Can you work these out from the model? Positions are in its coordinate system, mm. Face numbers are marked on the shaded views. A direction names the side the tool comes from. Coordinates: 2 decimals unless noted, no trailing zeros. Order: outer loops, then holes, each group sorted by start corner. A loop starts at its lowest first (then second) coordinate and runs counter-clockwise, first axis right, second up.
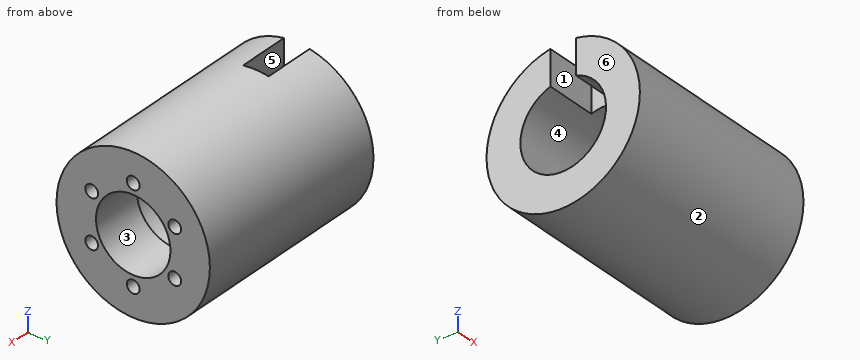
```python
from build123d import *

# Parameters (mm, degrees)
SKETCH1_W          = 25.4
SKETCH1_H          = 5.3975
SKETCH2_R          = 3.175
SKETCH2_R_2        = 18.5
CUT_EXTRUDE1_DEPTH = 25.4
CIRPATTERN1_COUNT  = 6
SKETCH3_W          = 25.4
SKETCH3_H          = 12.7
CUT_EXTRUDE2_DEPTH = 39.1


with BuildPart() as part:
    # Sketch1 → Revolve1 (revolve)
    with BuildSketch(Plane.XY):
        Polygon((-50.8, 38.1), (-50.8, 21.2725), (25.4, 21.2725), (50.8, 21.2725), (50.8, 38.1), (44.45, 38.1), align=None)
        with Locations((38.1, 18.57375)):
            Rectangle(SKETCH1_W, SKETCH1_H)
    revolve(axis=Axis((-50.8, 0, 0), (1, 0, 0)))

    # Sketch2 → Cut-Extrude1 (cut)
    with BuildSketch(Plane(origin=(50.8, 0, 0), x_dir=(0, 0, -1), z_dir=(1, 0, 0))):
        with Locations((-11.90625, -20.622229928)):
            Circle(SKETCH2_R)
        with Locations((11.90625, -20.622229928)):
            Circle(SKETCH2_R)
        with Locations((23.8125, 0)):
            Circle(SKETCH2_R)
        with Locations((11.90625, 20.622229928)):
            Circle(SKETCH2_R)
        with Locations((-11.90625, 20.622229928)):
            Circle(SKETCH2_R)
        Circle(SKETCH2_R_2)
    cut_extrude1 = extrude(amount=-CUT_EXTRUDE1_DEPTH, mode=Mode.SUBTRACT)

    # CirPattern1: Cut-Extrude1 ×6 about axis
    cirpattern1_axis = Axis((-50.8, 0, 0), (-1, 0, 0))
    for i in range(1, CIRPATTERN1_COUNT):
        add(cut_extrude1.rotate(cirpattern1_axis, i * 360 / CIRPATTERN1_COUNT), mode=Mode.SUBTRACT)

    # Sketch3 → Cut-Extrude2 (cut, through all)
    with BuildSketch(Plane.XY):
        with Locations((-38.1, 0)):
            Rectangle(SKETCH3_W, SKETCH3_H)
    extrude(amount=CUT_EXTRUDE2_DEPTH, mode=Mode.SUBTRACT)


solid = part.part
```
1. I'm going to push flat-ended pins straight in: pin 1 (10 mm diameter, centred on x = -33.5, z = 26, fed in from +Y); pin 2 (6 mm diameter, centred on x = -20, z = -6, fed in from -Y); pin 3 (8.5 mm diameter, centred on x = -40.5, z = 31, fed in from -Y). Where does each tip first touch, or does it pass through?
Completed:
pin 1: stops at y = 31.79
pin 2: stops at y = -37.98
pin 3: stops at y = -27.13
2. On a 3-axis mill with a long thin cutter (end or side, diameter ignored), from which of +Z, -Z, +X, -X, +Y, -Y can I reach the whole of each face in a straight line? I mean the marked faces 4, 5 and 6. Say none if no direction works.
Completed:
face 4: -X
face 5: +Z, -X
face 6: +Z, -Z, -X, +Y, -Y
3. Imagine slicing it at C-C on x = 45. Give the number of separate pieces and of enclosed holes in the cut face, then the cut area to 3 significant figures.
Completed:
separate pieces: 1
enclosed holes: 7
area: 3,300 mm2
4. Imagine slicing it at D-D on z = -16.5. Please give me the cut outline in (x, y).
Completed:
outline: (-50.8, -34.34) - (50.8, -34.34) - (50.8, -8.37) - (25.4, -8.37) - (25.4, -13.43) - (-50.8, -13.43) - close; (-50.8, 13.43) - (25.4, 13.43) - (25.4, 8.37) - (50.8, 8.37) - (50.8, 34.34) - (-50.8, 34.34) - close
5. Imagine slicing it at B-B on y = 0. Please give me the cut outline in (x, z).
Completed:
outline: (-50.8, -38.1) - (50.8, -38.1) - (50.8, -26.99) - (25.4, -26.99) - (25.4, -21.27) - (-50.8, -21.27) - close; (-25.4, 21.27) - (25.4, 21.27) - (25.4, 26.99) - (50.8, 26.99) - (50.8, 38.1) - (-25.4, 38.1) - close; (25.4, -20.64) - (50.8, -20.64) - (50.8, -18.5) - (25.4, -18.5) - close; (25.4, 18.5) - (50.8, 18.5) - (50.8, 20.64) - (25.4, 20.64) - close
6. Thinking about a two-plate mould opening in Z: for the marked faces 1, 2 and 3, which applies, pulls with the +Z half, pulls with the -Z half, needs draft (parallel to the pull), parting line crosses it, or undercut?
Completed:
face 1: needs draft
face 2: parting line crosses it
face 3: undercut
7. Please list where these lines run through material, in increasing order: probe 1 along Z at (x, y) = (40.5, 0); probe 2 along Y at (x, z) = (-17, 0); probe 3 along Y at (x, z) = (28, 11.5).
Completed:
probe 1: z = -38.1 to -26.99, -20.64 to -18.5, 18.5 to 20.64, 26.99 to 38.1
probe 2: y = -38.1 to -21.27, 21.27 to 38.1
probe 3: y = -36.32 to -23.77, -17.47 to -14.49, 14.49 to 17.47, 23.77 to 36.32
8. Imagine slicing it at A-A on z = 0. Please give me the cut outline in (x, y), then the cut area to 3 significant figures.
Completed:
outline: (-50.8, -38.1) - (50.8, -38.1) - (50.8, -18.5) - (25.4, -18.5) - (25.4, -21.27) - (-50.8, -21.27) - close; (-50.8, 21.27) - (25.4, 21.27) - (25.4, 18.5) - (50.8, 18.5) - (50.8, 38.1) - (-50.8, 38.1) - close
area: 3,560 mm2
